```python
from build123d import *

# Parameters (mm, degrees)
SKETCH1_W           = 69.8
SKETCH1_H           = 26
BOSS_EXTRUDE1_DEPTH = 20
FILLET1_R           = 13
SKETCH2_R           = 9.4
BOSS_EXTRUDE2_DEPTH = 1.2
SKETCH3_R           = 8.4
BOSS_EXTRUDE3_DEPTH = 2
CHAMFER1_SIZE       = 1
SKETCH4_R           = 7
SKETCH4_R_2         = 5
BOSS_EXTRUDE4_DEPTH = 6
SKETCH5_R           = 1.75
BOSS_EXTRUDE5_DEPTH = 5
CHAMFER2_SIZE       = 2.8
CUT_EXTRUDE1_START  = -1
SKETCH6_R           = 1.75
CUT_EXTRUDE1_DEPTH  = 1


with BuildPart() as part:
    # Sketch1 → Boss-Extrude1 (new body)
    with BuildSketch(Plane.XY):
        Rectangle(SKETCH1_W, SKETCH1_H)
    extrude(amount=BOSS_EXTRUDE1_DEPTH)

    # Fillet1
    fillet1_edges = [part.edges().sort_by_distance(p)[0] for p in [
        (-34.9, -13, 10),
        (-34.9, 13, 10),
        (34.9, -13, 10),
        (34.9, 13, 10),
    ]]
    fillet(fillet1_edges, radius=FILLET1_R - 0.0001)  # a hair under: the kernel refuses the full size

    # Sketch2 → Boss-Extrude2 (add)
    with BuildSketch(Plane.XY.offset(20)):
        Circle(SKETCH2_R)
    extrude(amount=BOSS_EXTRUDE2_DEPTH)

    # Sketch3 → Boss-Extrude3 (add)
    with BuildSketch(Plane.XY.offset(21.2)):
        Circle(SKETCH3_R)
    extrude(amount=BOSS_EXTRUDE3_DEPTH)

    # Chamfer1
    chamfer1_edges = [part.edges().sort_by_distance(p)[0] for p in [
        (-8.4, 0, 23.2),
    ]]
    chamfer(chamfer1_edges, length=CHAMFER1_SIZE)

    # Sketch4 → Boss-Extrude4 (add)
    with BuildSketch(Plane.XZ.offset(13)):
        with Locations(Location((0, 10, 0), (0, 0, 180))):
            Circle(SKETCH4_R)
        with Locations((0, 10)):
            Circle(SKETCH4_R_2, mode=Mode.SUBTRACT)
    extrude(amount=BOSS_EXTRUDE4_DEPTH)

    # Sketch5 → Boss-Extrude5 (add)
    with BuildSketch(Plane(origin=(0, 0, 0), x_dir=(-1, 0, 0), z_dir=(0, 0, -1))):
        with Locations(Location((-18.9, -8, 0), (0, 0, 180))):
            Circle(SKETCH5_R)
    extrude(amount=BOSS_EXTRUDE5_DEPTH)

    # Chamfer2
    chamfer2_edges = [part.edges().sort_by_distance(p)[0] for p in [
        (0, -13, 0),
        (0, 13, 0),
        (31.092417445, 9.192417445, 0),
        (31.092417445, -9.192417445, 0),
        (-31.092417445, 9.192417445, 0),
        (-31.092417445, -9.192417445, 0),
    ]]
    chamfer(chamfer2_edges, length=CHAMFER2_SIZE)

    # Sketch6 → Cut-Extrude1 (cut)
    with BuildSketch(Plane(origin=(0, 0, 0), x_dir=(-1, 0, 0), z_dir=(0, 0, -1)).offset(CUT_EXTRUDE1_START)):
        with BuildLine():
            Line((-21.4, -10.2), (-21.4, -8))
            ThreePointArc((-21.4, -8), (-18.9, -5.5), (-16.4, -8))
            Line((-16.4, -8), (-16.4, -10.2))
            Line((-16.4, -10.2), (-21.4, -10.2))
        make_face()
        with Locations((-18.9, -8)):
            Circle(SKETCH6_R, mode=Mode.SUBTRACT)
    extrude(amount=CUT_EXTRUDE1_DEPTH, mode=Mode.SUBTRACT)


solid = part.part
```
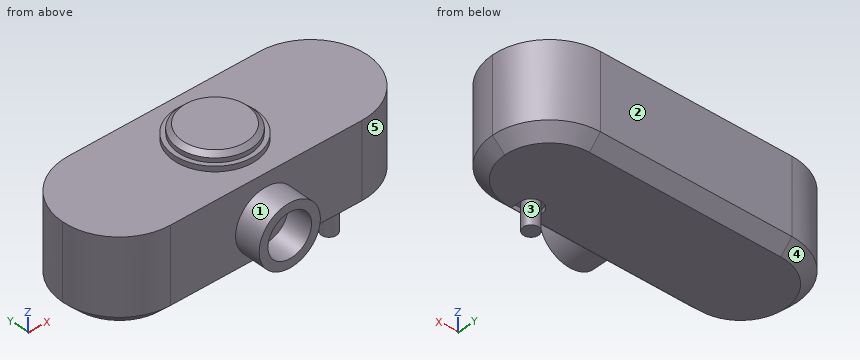
Input: part model. Units: mm. Frame: model coordinates. Face numbers are marked on the shaded views. A direction names the side the tool comes from. Coordinates: 2 decimals unless noted, no trailing zeros. Loops run counter-clockwise (first coordinate to the right, second up) from the corner with the lowest first, then second, coordinate; pieces in that order, holes last. Notation, with made-up numbers: (26, 74.5) - (36, 74.5) arc R13 cw to (36, 91.5) - close; hole circle Ø3 at (65, -39). An arc over 180 degrees is marked (long way). Answer in a Markdown table with one row per item.
(1) Set-up query: the marked faces 1 and 2. Return all of +Z, -Z, +X, -X, +Y, -Y with unobstructed straight access to the full face (end or side cutting, diameter ignored); none if empty.
Model answer:
| item | result |
|---|---|
| face 1 | -Y |
| face 2 | +Z, -Z, +X, -X, +Y |
(2) Material intervals for L1, parallel to Z at x = 0, y = -16.65; L2, parallel to Y at x = 12, z = 9.75; L3, parallel to X at y = -14.5, z = 9.5, sorted ascending. Write a range as from..to.
Model answer:
| item | result |
|---|---|
| L1 | z = 3..5, 15..17 |
| L2 | y = -13..13 |
| L3 | x = -6.98..-4.97, 4.97..6.98 |
(3) Cut plane A-A on x = 0. Output: boundary loops of the cut face in (y, z).
Model answer:
| item | result |
|---|---|
| outline | (-19, 3) - (-13, 3) - (-13, 2.8) - (-10.2, 0) - (10.2, 0) - (13, 2.8) - (13, 20) - (9.4, 20) - (9.4, 21.2) - (8.4, 21.2) - (8.4, 22.2) - (7.4, 23.2) - (-7.4, 23.2) - (-8.4, 22.2) - (-8.4, 21.2) - (-9.4, 21.2) - (-9.4, 20) - (-13, 20) - (-13, 17) - (-19, 17) - (-19, 15) - (-13, 15) - (-13, 5) - (-19, 5) - close |
(4) Mould query, pull axis X, two halves, no side actions, for the marked faces 3, 4 and 5. Classes: pulls with the +X half, pulls with the -X half, needs draft (parallel to the pull), parting line crosses it, or undercut.
Model answer:
| item | result |
|---|---|
| face 3 | undercut |
| face 4 | pulls with the -X half |
| face 5 | pulls with the +X half |
(5) Cut plane C-C on x = 18.9. Output: boundary loops of the cut face in (y, z).
Model answer:
| item | result |
|---|---|
| outline | (-13, 2.8) - (-10.2, 0) - (-10.2, 1) - (-9.75, 1) - (-9.75, -5) - (-6.25, -5) - (-6.25, 1) - (-5.5, 1) - (-5.5, 0) - (10.2, 0) - (13, 2.8) - (13, 20) - (-13, 20) - close |
(6) Pin query (flat end, axial travel): P1, Ø8, axis at x = 17, y = 2.5, coming from the +Z side; P2, Ø8, axis at x = 17.5, z = 19.5, coming from the -Y side; P3, Ø5, axis at y = 4, z = 4.5, coming from the +X side. Return the tip coordinate at first contact, or that it passes through.
Model answer:
| item | result |
|---|---|
| P1 | stops at z = 20 |
| P2 | stops at y = -13 |
| P3 | stops at x = 34.81 |
